Verification items for this drawing (mm, ordinates from the low corner). Coordinates: 2 decimals unless noted, no trailing zeros. Write each loop counter-clockwise with the first axis right and the second up, starting at its lowest first coordinate (ties: lowest second). Pieces come first, ordered by that corner, then holes. Notation, with made-up numbers: (13, 7) -> (48, 7) arc R31 ccw to (48, 33) -> close; hole circle Ø11 at (-28.5, 12). An arc over 180 degrees is marked (long way). Answer as CSV lines item,"result".
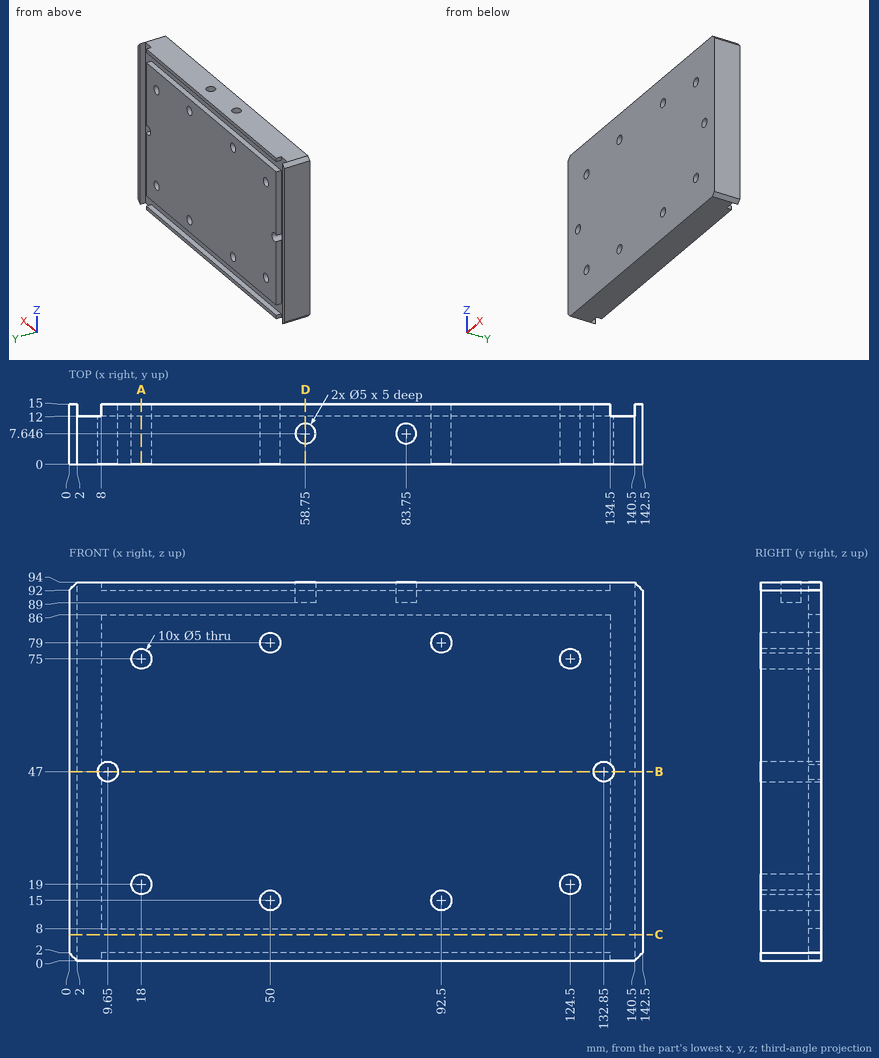
Item 1: Cross-section at D-D, the plane x = 58.75. Record the cut outline in (y, z), plus the area to 3 significant figures.
Responses:
outline,"(0, 0) -> (15, 0) -> (15, 2) -> (12, 2) -> (12, 8) -> (15, 8) -> (15, 86) -> (12, 86) -> (12, 92) -> (15, 92) -> (15, 94) -> (10.15, 94) -> (10.15, 89) -> (5.15, 89) -> (5.15, 94) -> (0, 94) -> close"
area,"1,350 mm2"
Item 2: Thickness scan on probe 1 along X at (y, z) = (11, 15); probe 2 along Z at (x, y) = (38, 14); probe 3 along X at (y, z) = (9.5, 75). Record the ranges inside material, lowest first.
Responses:
probe 1,"x = 0 to 47.5, 52.5 to 90, 95 to 142.5"
probe 2,"z = 0 to 2, 8 to 86, 92 to 94"
probe 3,"x = 0 to 15.5, 20.5 to 122, 127 to 142.5"
Item 3: Depth check by flat-ended pin: pin 1 Ø1.6 at (y, z) = (13, 93) entering from -X; pin 2 Ø3 at (x, z) = (50, 79) entering from -Y; pin 3 Ø4 at (x, y) = (58.75, 7.65) entering from +Z; pin 4 Ø0.6 at (y, z) = (13.5, 93) entering from +X. Enter the tip coordinate at first touch or a pass-through.
Responses:
pin 1,"stops at x = 0.2"
pin 2,"passes through"
pin 3,"stops at z = 89"
pin 4,"stops at x = 141.8"
Item 4: Cross-section at A-A, the plane x = 18. Record the cut outline in (y, z).
Responses:
outline,"(0, 0) -> (15, 0) -> (15, 2) -> (12, 2) -> (12, 8) -> (15, 8) -> (15, 16.5) -> (0, 16.5) -> close; (0, 21.5) -> (15, 21.5) -> (15, 72.5) -> (0, 72.5) -> close; (0, 77.5) -> (15, 77.5) -> (15, 86) -> (12, 86) -> (12, 92) -> (15, 92) -> (15, 94) -> (0, 94) -> close"
Item 5: Cross-section at C-C, the plane z = 6.5. Record the cut outline in (x, y).
Responses:
outline,"(0, 0) -> (142.5, 0) -> (142.5, 15) -> (140.5, 15) -> (140.5, 12) -> (2, 12) -> (2, 15) -> (0, 15) -> close"
Item 6: Cross-section at B-B, the plane z = 47. Record the cut outline in (x, y), plus the area to 3 significant figures.
Responses:
outline,"(0, 0) -> (7.15, 0) -> (7.15, 12) -> (2, 12) -> (2, 15) -> (0, 15) -> close; (12.15, 0) -> (130.35, 0) -> (130.35, 15) -> (12.15, 15) -> close; (135.35, 0) -> (142.5, 0) -> (142.5, 15) -> (140.5, 15) -> (140.5, 12) -> (135.35, 12) -> close"
area,"1,960 mm2"
